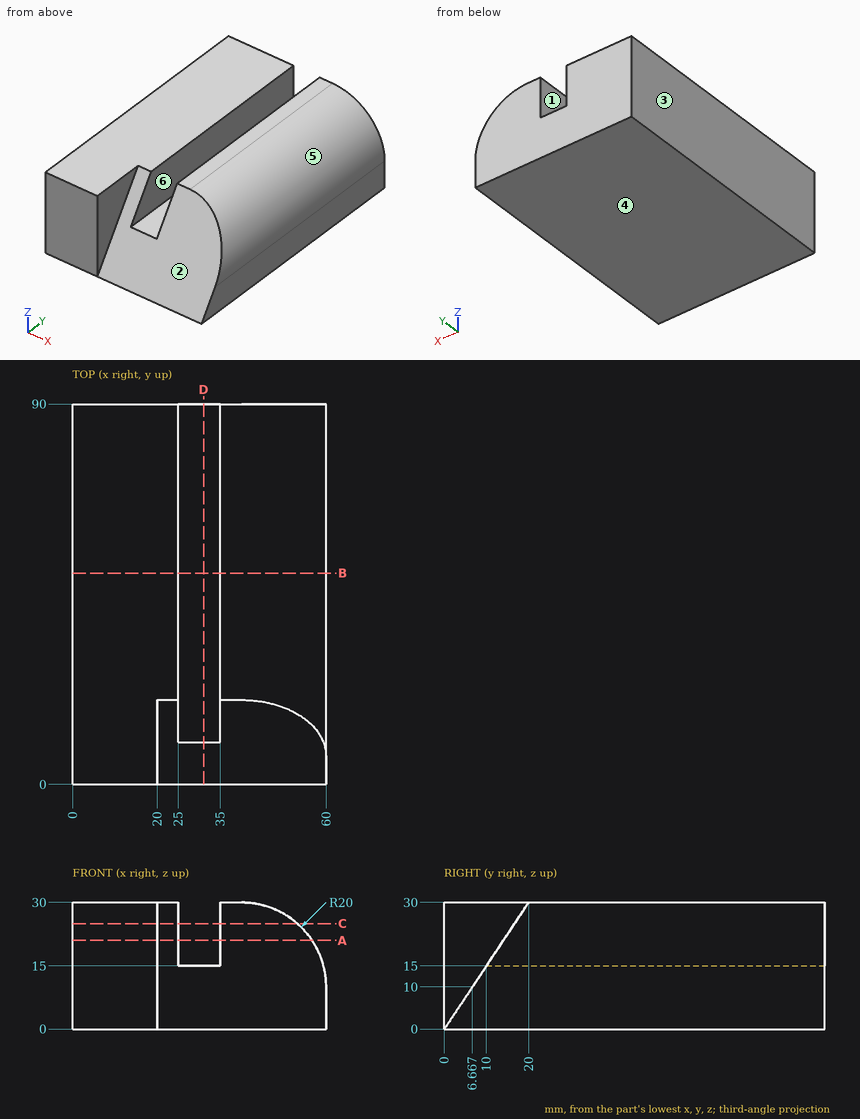
Here's the drawing with two shaded views (mm, measured from the low corner). I have some questions. A direction names the side the tool comes from. Give positions to 0.01 mm unless a question says otherwise; leave off trailing zeros. Loops run counter-clockwise (first coordinate to the right, second up) from the corner with the lowest first, then second, coordinate; pieces in that order, holes last. Notation, with made-up numbers: M 71.25,18.5 L 112.25,18.5 A29 cw 112.25,45.5 Z; hole C 2.5,63 d8. An arc over 180 degrees is marked long. One line per item, written item: value.
(1) Suppose I cut it at A-A on z = 21. List the corners of the cut face in (x, y) for me, plus the area to 3 significant figures.
Returned:
outline: M 0,0 L 20,0 L 20,14 L 25,14 L 25,90 L 0,90 Z; M 35,14 L 56.7,14 L 56.7,90 L 35,90 Z
area: 3,830 mm^2
(2) Suppose I cut it at C-C on z = 25. List the corners of the cut face in (x, y) for me, plus the area to 3 significant figures.
Returned:
outline: M 0,0 L 20,0 L 20,16.67 L 25,16.67 L 25,90 L 0,90 Z; M 35,16.67 L 53.23,16.67 L 53.23,90 L 35,90 Z
area: 3,500 mm^2
(3) We'd pull the mould along X, two halves only. Please class the marked faces 4, 5 and 6: released by +X, released by -X, zero draft, split by the parting line, or undercut.
Returned:
face 4: zero draft
face 5: released by +X
face 6: undercut
(4) Suppose I cut it at B-B on y = 50. List the corners of the cut face in (x, z) for me, plus the area to 3 significant figures.
Returned:
outline: M 0,0 L 60,0 L 60,10 A20 ccw 40,30 L 35,30 L 35,15 L 25,15 L 25,30 L 0,30 Z
area: 1,560 mm^2
(5) I need wall thicknesses on line 1 (Z direction, x = 32.5, y = 77); line 2 (X direction, y = 86, z = 27) (1 decimal); line 3 (X direction, y = 54, z = 26). Which ranges of each line are inside material? Lowest first, please.
Returned:
line 1: 0 to 15
line 2: 0 to 25, 35 to 50.5
line 3: 0 to 25, 35 to 52
(6) Suppose I cut it at D-D on x = 31. List the corners of the cut face in (y, z) for me, plus the area to 4 significant figures.
Returned:
outline: M 0,0 L 90,0 L 90,15 L 10,15 Z
area: 1,275 mm^2
(7) Which directions (+Z, -Z, +X, -X, +Y, -Y) give clear straight access to the entire face, cutting with the end or side of a thin tool? Please do the marked faces 1, 2 and 3.
Returned:
face 1: +Z, +Y, -Y
face 2: +Z, +X, -Y
face 3: +Z, -Z, -X, +Y, -Y
(8) Will these pins go through, and if not, where does the flat tip stop? pin 1 (10 mm diameter, centred on x = 37, z = 13, fed in from -Y); pin 2 (3 mm diameter, centred on y = 47, z = 16, fed in from +X); pin 3 (5 mm diameter, centred on x = 31.5, y = 36, fed in from +Z).
Returned:
pin 1: y = 5.33
pin 2: x = 59.49
pin 3: z = 15
